Can you work these out from the model? Positions are in its coordinate system, mm. Face numbers are marked on the shaded views. Give positions to 0.01 mm unless a question says otherwise; leave off trailing zeros. Order: outer loops, then holes, each group sorted by start corner. A loop starts at its lowest first (then second) coordinate and runs counter-clockwise, first axis right, second up.
Item 1: I want a section at B-B, the plane z = 39. Write out the boundary of the cut face in (x, y).
Item 2: I want a section at C-C, the plane z = 243. Write out the boundary of the cut face in (x, y), then the cut area to 3 significant figures.
Item 3: If I drill on line 1 along Z through (x, y) = (-30, 20); line 2 along Y through (x, z) = (61.5, 413); line 3 along X through (y, z) = (28, 291), over which ranges is the centre line in solid material (lowest first)?
Item 4: I want a section at D-D, the plane x = 139. Write out the boundary of the cut face in (y, z).
Item 5: I'm going to push flat-ended pins straight in: pin 1 Ø1.5 at (x, y) = (-30, 14.5) entering from -Z; pin 2 Ø2.5 at (x, y) = (-30, 15.5) entering from +Z; pin 3 Ø2.5 at (x, y) = (-30, 55) entering from +Z. Where does each tip first touch, or does it pass through?
Item 6: If we mould it in two halves opening along X, with no side actions, what happens to the marked faces 1, 2 and 3? For each: +X half, -X half, draft (parallel to the pull), parting line (faces both ways), or undercut.
Item 7: I want a section at A-A, the plane y = 20. Write out the boundary of the cut face in (x, z).
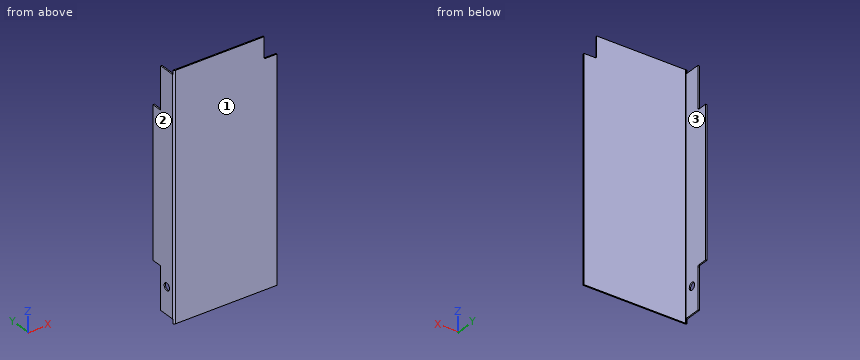
```python
from build123d import *

# Parameters (mm, degrees)
BASE_FLANGE1_DEPTH       = 570
CUT_EXTRUDE1_OUTLINE_W   = 3
CUT_EXTRUDE1_OUTLINE_H   = 25
CUT_EXTRUDE1_DEPTH       = 107
CUT_EXTRUDE1_START       = 463
CUT_EXTRUDE1_2_OUTLINE_W = 3
CUT_EXTRUDE1_2_OUTLINE_H = 25
CUT_EXTRUDE1_2_DEPTH     = 107
CUT_EXTRUDE1_START_2     = -32
CUT_EXTRUDE1_3_DEPTH     = 5
CUT_EXTRUDE1_START_3     = -1
CUT_EXTRUDE1_4_DEPTH     = 11
CUT_EXTRUDE1_START_4     = 560
CUT_EXTRUDE1_5_DEPTH     = 11
CUT_EXTRUDE3_REACH       = 613.523
CUT_EXTRUDE4_REACH       = 623.872
SKETCH8_R                = 8.75


with BuildPart() as part:
    # Base-Flange1: sheet metal written as solids
    # Sketch1 → Base-Flange1 (new body)
    with BuildSketch(Plane.XY):
        with BuildLine():
            Line((-28.256118786, 65), (-28.256118786, 0.7366))
            ThreePointArc((-28.256118786, 0.7366), (-28.040373641, 0.215745145), (-27.519518786, 0))
            Line((-27.519518786, 0), (211.743881214, 0))
            Line((211.743881214, 0), (211.743881214, -3))
            Line((211.743881214, -3), (-27.519518786, -3))
            ThreePointArc((-27.519518786, -3), (-30.161693985, -1.905575199), (-31.256118786, 0.7366))
            Line((-31.256118786, 0.7366), (-31.256118786, 65))
            Line((-31.256118786, 65), (-28.256118786, 65))
        make_face()
    extrude(amount=BASE_FLANGE1_DEPTH)

    # Cut-Extrude1: read off the stored shape, not the designer's step
    # Cut-Extrude1 outline → Cut-Extrude1 (cut)
    with BuildSketch(Plane.XY):
        with Locations((-29.756118786, 52.5)):
            Rectangle(CUT_EXTRUDE1_OUTLINE_W, CUT_EXTRUDE1_OUTLINE_H)
    extrude(amount=CUT_EXTRUDE1_DEPTH, mode=Mode.SUBTRACT)

    # Cut-Extrude1 2 outline → Cut-Extrude1 2 (cut)
    with BuildSketch(Plane.XY.offset(CUT_EXTRUDE1_START)):
        with Locations((-29.756118786, 52.5)):
            Rectangle(CUT_EXTRUDE1_2_OUTLINE_W, CUT_EXTRUDE1_2_OUTLINE_H)
    extrude(amount=CUT_EXTRUDE1_2_DEPTH, mode=Mode.SUBTRACT)

    # Cut-Extrude1 3 outline → Cut-Extrude1 3 (cut)
    with BuildSketch(Plane.YZ.offset(CUT_EXTRUDE1_START_2)):
        with BuildLine():
            Line((65, 110), (43, 110))
            ThreePointArc((43, 110), (40.878679656, 109.121320344), (40, 107))
            Line((40, 107), (65, 107))
            Line((65, 107), (65, 110))
        make_face()
        with BuildLine():
            Line((43, 460), (65, 460))
            Line((65, 460), (65, 463))
            Line((65, 463), (40, 463))
            ThreePointArc((40, 463), (40.878679656, 460.878679656), (43, 460))
        make_face()
    extrude(amount=CUT_EXTRUDE1_3_DEPTH, mode=Mode.SUBTRACT)

    # Cut-Extrude1 4 outline → Cut-Extrude1 4 (cut)
    with BuildSketch(Plane.XY.offset(CUT_EXTRUDE1_START_3)):
        with BuildLine():
            Line((-31.182796008, 0), (-28.241664587, 0.591393245))
            ThreePointArc((-28.241664587, 0.591393245), (-28.252496329, 0.663637809), (-28.256118786, 0.7366))
            Line((-28.256118786, 0.7366), (-28.256118786, 40))
            Line((-28.256118786, 40), (-31.256118786, 40))
            Line((-31.256118786, 40), (-31.256118786, 0.7366))
            ThreePointArc((-31.256118786, 0.7366), (-31.237742907, 0.36647982), (-31.182796008, 0))
        make_face()
    extrude(amount=CUT_EXTRUDE1_4_DEPTH, mode=Mode.SUBTRACT)

    # Cut-Extrude1 5 outline → Cut-Extrude1 5 (cut)
    with BuildSketch(Plane.XY.offset(CUT_EXTRUDE1_START_4)):
        with BuildLine():
            Line((-31.182796008, 0), (-28.241664587, 0.591393245))
            ThreePointArc((-28.241664587, 0.591393245), (-28.252496329, 0.663637809), (-28.256118786, 0.7366))
            Line((-28.256118786, 0.7366), (-28.256118786, 40))
            Line((-28.256118786, 40), (-31.256118786, 40))
            Line((-31.256118786, 40), (-31.256118786, 0.7366))
            ThreePointArc((-31.256118786, 0.7366), (-31.237742907, 0.36647982), (-31.182796008, 0))
        make_face()
    extrude(amount=CUT_EXTRUDE1_5_DEPTH, mode=Mode.SUBTRACT)

    # Sketch7 → Cut-Extrude3 (cut, up to next)
    with BuildSketch(Plane(origin=(0, 0, 0), x_dir=(1, 0, 0), z_dir=(0, 1, 0)), mode=Mode.PRIVATE) as cut_extrude3_sk1:
        with BuildLine():
            Line((211.743881214, -520), (184.743881214, -520))
            ThreePointArc((184.743881214, -520), (182.62256087, -520.878679656), (181.743881214, -523))
            Line((181.743881214, -523), (181.743881214, -570))
            Line((181.743881214, -570), (211.743881214, -570))
            Line((211.743881214, -570), (211.743881214, -520))
        make_face()
    cut_extrude3_tool1 = extrude(cut_extrude3_sk1.sketch, amount=-CUT_EXTRUDE3_REACH, mode=Mode.PRIVATE) & part.part
    add(cut_extrude3_tool1.solids().sort_by_distance((196.762356, 0, 545.031368))[0], mode=Mode.SUBTRACT)

    # Sketch8 → Cut-Extrude4 (cut, up to next)
    with BuildSketch(Plane(origin=(-28.256118786, 0, 0), x_dir=(0, 0, -1), z_dir=(1, 0, 0)), mode=Mode.PRIVATE) as cut_extrude4_sk1:
        with Locations(Location((-73.034040989, 20, 0), (0, 0, 90))):
            Circle(SKETCH8_R)
    cut_extrude4_tool1 = extrude(cut_extrude4_sk1.sketch, amount=-CUT_EXTRUDE4_REACH, mode=Mode.PRIVATE) & part.part
    add(cut_extrude4_tool1.solids().sort_by_distance((-28.256119, 20, 73.034041))[0], mode=Mode.SUBTRACT)


solid = part.part
```
Results list:
1. outline: (-31.26, 0.74) arc R3.74 ccw to (-27.52, -3) - (211.74, -3) - (211.74, 0) - (-27.52, 0) arc R0.74 cw to (-28.26, 0.74) - (-28.26, 40) - (-31.26, 40) - close
2. outline: (-31.26, 0.74) arc R3.74 ccw to (-27.52, -3) - (211.74, -3) - (211.74, 0) - (-27.52, 0) arc R0.74 cw to (-28.26, 0.74) - (-28.26, 65) - (-31.26, 65) - close
2. area: 921 mm2
3. line 1: z = 10 to 64.28, 81.78 to 560
3. line 2: y = -3 to 0
3. line 3: x = -31.26 to -28.26
4. outline: (-3, 0) - (0, 0) - (0, 570) - (-3, 570) - close
5. pin 1: stops at z = 10
5. pin 2: stops at z = 560
5. pin 3: stops at z = 460
6. face 1: draft
6. face 2: -X half
6. face 3: +X half
7. outline: (-31.26, 10) - (-28.26, 10) - (-28.26, 64.28) - (-31.26, 64.28) - close; (-31.26, 81.78) - (-28.26, 81.78) - (-28.26, 560) - (-31.26, 560) - close
